from build123d import *

# Parameters (mm, degrees)
SKETCH_R     = 8.5
SKETCH_R_2   = 7
PAD_DEPTH    = 6.5
SKETCH001_R  = 3
PAD001_DEPTH = 4.8
PAD002_DEPTH = 8.5
SKETCH003_R  = 6
PAD003_DEPTH = 2
SKETCH004_W  = 12
SKETCH004_H  = 3
PAD004_DEPTH = 2
SKETCH005_W  = 27.5
SKETCH005_H  = 3
PAD005_DEPTH = 7
SKETCH006_R  = 2.75
PAD006_DEPTH = 28
SKETCH007_R  = 7
PAD007_DEPTH = 14
SKETCH008_R  = 7
PAD008_DEPTH = 14


with BuildPart() as part:
    # Sketch → Pad (new body)
    with BuildSketch(Plane.XY):
        Circle(SKETCH_R)
        Circle(SKETCH_R_2, mode=Mode.SUBTRACT)
    extrude(amount=PAD_DEPTH)

    # Sketch001 (on Face4 of Pad) → Pad001 (join)
    with BuildSketch(Plane.XY.offset(6.5)):
        with BuildLine():
            ThreePointArc((2.6404501177, -16.3733937587), (10.7, -18.532943641), (12.8595498823, -10.4733937587))
            Line((12.8595498823, -10.4733937587), (8.1689615905, -2.3490565198))
            ThreePointArc((-2.0501381742, -8.2490565198), (4.25, -7.3612159322), (8.1689615905, -2.3490565198))
            Line((2.6404501177, -16.3733937587), (-2.0501381742, -8.2490565198))
        make_face()
        with Locations((7.75, -13.4233937587)):
            Circle(SKETCH001_R, mode=Mode.SUBTRACT)
    extrude(amount=-PAD001_DEPTH)

    # Sketch002 (on Face3 of Pad001) → Pad002 (join)
    with BuildSketch(Plane.XY.offset(6.5)):
        with BuildLine():
            Line((0, 10.8), (9.8, 10.8))
            ThreePointArc((13.7613854943, 4.8274495625), (13.3834317966, 8.8767659875), (9.8, 10.8))
            Line((9.9495263577, -4.2008243546), (13.7613854943, 4.8274495625))
            ThreePointArc((0, -10.8), (5.9695517826, -9.000247303), (9.9495263577, -4.2008243546))
            Line((0, -10.8), (-9.8000000001, -10.8))
            ThreePointArc((-13.7613854943, -4.8274495625), (-13.3834317966, -8.8767659875), (-9.8000000001, -10.8))
            Line((-9.9495263577, 4.2008243546), (-13.7613854943, -4.8274495625))
            ThreePointArc((7e-10, 10.8), (-5.9695517823, 9.0002473032), (-9.9495263577, 4.2008243546))
        make_face()
    extrude(amount=PAD002_DEPTH)

    # Sketch003 (on Face20 of Pad002) → Pad003 (join)
    with BuildSketch(Plane.XY.offset(15)):
        Circle(SKETCH003_R)
    extrude(amount=PAD003_DEPTH)

    # Sketch004 (on Face22 of Pad003) → Pad004 (join)
    with BuildSketch(Plane.XY.offset(17)):
        Rectangle(SKETCH004_W, SKETCH004_H)
    extrude(amount=PAD004_DEPTH)

    # Sketch005 (on Face32 of Pad004) → Pad005 (join)
    with BuildSketch(Plane.XY.offset(19)):
        with Locations((-7.75, 0)):
            Rectangle(SKETCH005_W, SKETCH005_H)
    extrude(amount=PAD005_DEPTH)

    # Sketch006 → Pad006 (join, symmetric)
    with BuildSketch(Plane.YZ):
        with Locations((0, 5)):
            Circle(SKETCH006_R)
    extrude(amount=PAD006_DEPTH, both=True)

    # Sketch007 (on Face13 of Pad006) → Pad007 (join)
    with BuildSketch(Plane.YZ.offset(28)):
        with Locations((0, 5)):
            Circle(SKETCH007_R)
    extrude(amount=-PAD007_DEPTH)

    # Sketch008 (on Face20 of Pad007) → Pad008 (join)
    with BuildSketch(Plane(origin=(-28, 0, 0), x_dir=(0, -1, 0), z_dir=(-1, 0, 0))):
        with Locations((0, 5)):
            Circle(SKETCH008_R)
    extrude(amount=-PAD008_DEPTH)


solid = part.part
CAD build for the part. Positions are in the model's coordinates, mm. A direction names the side the tool comes from. Give positions to 0.01 mm unless a question says otherwise; leave off trailing zeros. Write each loop counter-clockwise with the first axis right and the second up, starting at its lowest first coordinate (ties: lowest second). Pieces come first, ordered by that corner, then holes. Notation, with made-up numbers: (50.25, -3) -> (79.25, -3) arc R30 ccw to (79.25, 34) -> close; hole circle Ø7 at (24.25, 73). An arc over 180 degrees is marked (long way). Return JSON: item names as keys, results as strings.
Item 1: Band-saw the part on C-C (z = 4.25). List the corners of the cut face in (x, y).
Answer below:
{"outline": "(-28, -6.96) -> (-14, -6.96) -> (-14, -2.65) -> (-8.08, -2.65) arc R8.5 ccw to (-2.05, -8.25) -> (2.64, -16.37) arc R5.9 ccw to (12.86, -10.47) -> (8.34, -2.65) -> (14, -2.65) -> (14, -6.96) -> (28, -6.96) -> (28, 6.96) -> (14, 6.96) -> (14, 2.65) -> (8.08, 2.65) arc R8.5 ccw to (-8.08, 2.65) -> (-14, 2.65) -> (-14, 6.96) -> (-28, 6.96) -> close; hole (-6.48, -2.65) arc R7 ccw to (6.48, -2.65) -> close; hole (-6.48, 2.65) -> (6.48, 2.65) arc R7 ccw to start; hole circle Ø6 at (7.75, -13.42)"}
Item 2: Band-saw the part on B-B (y = -14). List the corners of the cut face in (x, z), then the cut area to 3 significant figures.
Answer below:
{"outline": "(1.27, 1.7) -> (4.81, 1.7) -> (4.81, 6.5) -> (1.27, 6.5) -> close; (10.69, 1.7) -> (13.62, 1.7) -> (13.62, 6.5) -> (10.69, 6.5) -> close", "area": "31.0 mm2"}
Item 3: Two-plate mould, pull along X, no slides. Class faces 1 (the cylindrical face through (21.098, 3.763, 10.902)), 2 (the flat face through (0.33, -12.37, 4.13)), 3 (the cylindrical face through (0.1, -0.08, 2.25)): +X half, -X half, draft (parallel to the pull), parting line (faces both ways), or undercut.
Answer below:
{"face 1": "draft", "face 2": "-X half", "face 3": "undercut"}
Item 4: Band-saw the part on A-A (x = -19). List the corners of the cut face in (y, z).
Answer below:
{"outline": "circle Ø14 at (0, 5); (-1.5, 19) -> (1.5, 19) -> (1.5, 26) -> (-1.5, 26) -> close"}
Item 5: Drill centre lines: probe 1 along X at (y, z) = (3, 1.25); probe 2 along Y at (x, z) = (0, 4.75); probe 3 along X at (y, z) = (1, 11.5). Where is each one in solid material? Low to high.
Answer below:
{"probe 1": "x = -28 to -14, -7.95 to -6.32, 6.32 to 7.95, 14 to 28", "probe 2": "y = -11.8 to -7, -2.74 to 2.74, 7 to 8.5", "probe 3": "x = -28 to -14, -11.3 to 12.15, 14 to 28"}
Item 6: Band-saw the part on D-D (x = 15). List the corners of the cut face in (y, z), then the cut area to 3 significant figures.
Answer below:
{"outline": "circle Ø14 at (0, 5)", "area": "154 mm2"}
Item 7: Tool access for faces 4 (the cylindrical face through (11.725, -0.596, 2.315)), 5 (the flat face through (-14, 0, 19)), 6 (the flat face through (-21.5, 0, 22)), 7 (the flat face through (6, 0, 21)): list every direction of +Z, -Z, +X, -X, +Y, -Y with a clear straight run to the whole face (end or side of a thin tool).
Answer below:
{"face 4": "none", "face 5": "-X, +Y, -Y", "face 6": "+Z, -X, +Y, -Y", "face 7": "+Z, +X, +Y, -Y"}
Item 8: Drop flat-ended pins along their axis: pin 1 (2 mm diameter, centred on x = -4.5, y = 3, fed in from +Z); pin 2 (5.5 mm diameter, centred on x = 7.75, y = -13.42, fed in from -Z); pin 3 (2 mm diameter, centred on y = -4, z = 17, fed in from -X); pin 4 (3.5 mm diameter, centred on y = 0.5, z = 20.5, fed in from +X). Give the stop position or say it passes through.
Answer below:
{"pin 1": "stops at z = 17", "pin 2": "passes through", "pin 3": "stops at x = -5.2", "pin 4": "stops at x = 6"}
